```python
from build123d import *

# Parameters (mm, degrees)
F0_W     = 25.4
F0_H     = 593.5472
F0_W_2   = 593.5345
F0_H_2   = 25.4
F1_DEPTH = 25.4
F2_W     = 5.08
F2_H     = 583.3872
F3_DEPTH = 7.62
F4_W     = 583.3745
F4_H     = 5.08
F5_DEPTH = 7.62


with BuildPart() as f1:
    # F0 (on Front) → F1 (new body)
    with BuildSketch(Plane.XZ):
        with Locations((101.022233, 190.518868)):
            Rectangle(F0_W, F0_H)
        Polygon((88.322233, -106.254732), (88.322233, -131.654732), (113.722233, -106.254732), align=None)
        with Locations((-208.445017, -118.954732)):
            Rectangle(F0_W_2, F0_H_2)
    extrude(amount=F1_DEPTH)

    # F2 (on face) → F3 (cut)
    with BuildSketch(Plane(origin=(0, 0, 0), x_dir=(-1, 0, 0), z_dir=(0, 1, 0))):
        with Locations((-101.022233, 185.438868)):
            Rectangle(F2_W, F2_H)
    extrude(amount=-F3_DEPTH, mode=Mode.SUBTRACT)

    # F4 (on face) → F5 (cut)
    with BuildSketch(Plane(origin=(0, 0, 0), x_dir=(-1, 0, 0), z_dir=(0, 1, 0))):
        with Locations((203.365017, -118.954732)):
            Rectangle(F4_W, F4_H)
    extrude(amount=-F5_DEPTH, mode=Mode.SUBTRACT)


solid = f1.part
```
For this review, take the finished solid that the model builds, in its own axes (mm). A direction names the side the tool comes from. Give positions to 0.01 mm unless a question says otherwise; leave off trailing zeros. Write each loop counter-clockwise with the first axis right and the second up, starting at its lowest first coordinate (ties: lowest second). Pieces come first, ordered by that corner, then holes.
Item 1: Wall thickness on probe 1 along Z at (x, y) = (-149, -4.75); probe 2 along X at (y, z) = (-3, -77); probe 3 along X at (y, z) = (-8.25, 263): over which ranges is each line inside the solid? List them lowest first.
Item 2: Take a section at A-A (x = 33.5). Give the boundary of the cut face in (y, z).
Item 3: Take a section at B-B (y = -14.5). Give the boundary of the cut face in (x, z), and give its area (3 significant figures).
Item 4: Machinability: for faces 1 (the face through (-213, -13, -131.655)), 2 (the face through (-213, -13, -106.255)), which of the approach directions +Z, -Z, +X, -X, +Y, -Y give a long, thin tool a straight path to every point of the face, cutting with its end or side? Answer none if there is none.
Item 5: Insertion check: P1, Ø4, axis at x = 100, z = 264.5, coming from the +Y side; P2, Ø2.5, axis at x = -224, y = -5.5, coming from the +Z side; P3, Ø12, axis at y = -7.5, z = 382.5, coming from the -X side; P4, Ø2.5, axis at y = -3, z = -118, coming from the +X side. Each pin has a flat end and moves straight along its axis. Give the tip position at first contact, or say it passes through.
Item 6: Take a section at C-C (z = 216.5). Give the boundary of the cut face in (x, y), and give its area (3 significant figures).
Established:
1. probe 1: z = -131.65 to -121.49, -116.41 to -106.25
1. probe 2: x = 88.32 to 98.48, 103.56 to 113.72
1. probe 3: x = 88.32 to 113.72
2. outline: (-25.4, -131.65) - (0, -131.65) - (0, -121.49) - (-7.62, -121.49) - (-7.62, -116.41) - (0, -116.41) - (0, -106.25) - (-25.4, -106.25) - close
3. outline: (-505.21, -131.65) - (88.32, -131.65) - (113.72, -106.25) - (113.72, 487.29) - (88.32, 487.29) - (88.32, -106.25) - (-505.21, -106.25) - close
3. area: 30,500 mm2
4. face 1: -Z, +X, -X, +Y, -Y
4. face 2: +Z, -X, +Y, -Y
5. P1: stops at y = 0
5. P2: stops at z = -106.25
5. P3: stops at x = 88.32
5. P4: stops at x = 103.23
6. outline: (88.32, -25.4) - (113.72, -25.4) - (113.72, 0) - (103.56, 0) - (103.56, -7.62) - (98.48, -7.62) - (98.48, 0) - (88.32, 0) - close
6. area: 606 mm2
